from build123d import *

# Parameters (mm, degrees)
ESBO_O1_R                     = 7.5
RESSALTO_EXTRUS_O1_DEPTH      = 95
CORTE_EXTRUS_O1_START         = -7.5
ESBO_O2_R                     = 7.5
ESBO_O2_R_2                   = 6.5
CORTE_EXTRUS_O1_DEPTH         = 7.5
FILETE1_R                     = 5
FURO_ROSCADO_DE_M6X1_01_D     = 5
FURO_ROSCADO_DE_M6X1_01_DEPTH = 15.497848452
FURO_ROSCADO_DE_M6X1_01_TIP   = 1.502151548
CHANFRO1_SIZE                 = 0.5
CORTE_EXTRUS_O2_DEPTH         = 96.590271472
CORTE_EXTRUS_O2_DEPTH_BACK    = 96.590271472
ESBO_O8_W                     = 1
ESBO_O8_H                     = 50


with BuildPart() as part:
    # Esboço1 → Ressalto-extrusão1 (new, symmetric)
    with BuildSketch(Plane.XY):
        Circle(ESBO_O1_R)
    extrude(amount=RESSALTO_EXTRUS_O1_DEPTH, both=True)

    # Esboço2 → Corte-extrusão1 (cut)
    with BuildSketch(Plane(origin=(0, 0, -95), x_dir=(-1, 0, 0), z_dir=(0, 0, -1)).offset(CORTE_EXTRUS_O1_START)):
        Circle(ESBO_O2_R)
        Circle(ESBO_O2_R_2, mode=Mode.SUBTRACT)
    extrude(amount=CORTE_EXTRUS_O1_DEPTH, mode=Mode.SUBTRACT)

    # Filete1
    filete1_edges = [part.edges().sort_by_distance(p)[0] for p in [
        (-7.5, 0, 95),
    ]]
    fillet(filete1_edges, radius=FILETE1_R)

    # Furo roscado de M6x1.01
    with Locations(Plane(origin=(0, 0, -95), x_dir=(-1, 0, 0), z_dir=(0, 0, -1))):
        with Locations((0, 0)):
            Hole(FURO_ROSCADO_DE_M6X1_01_D / 2, depth=FURO_ROSCADO_DE_M6X1_01_DEPTH)
            with Locations((0, 0, -(FURO_ROSCADO_DE_M6X1_01_DEPTH + FURO_ROSCADO_DE_M6X1_01_TIP / 2))):  # 118° drill point
                Cone(0, FURO_ROSCADO_DE_M6X1_01_D / 2, FURO_ROSCADO_DE_M6X1_01_TIP, mode=Mode.SUBTRACT)

    # Chanfro1
    chanfro1_edges = [part.edges().sort_by_distance(p)[0] for p in [
        (6.5, 0, -95),
    ]]
    chamfer(chanfro1_edges, length=CHANFRO1_SIZE)

    # Esboço8 → Corte-extrusão2 (cut, two sides: drawn at the far end of the back side and taken through both)
    with BuildSketch(Plane(origin=(0, 0, 0), x_dir=(1, 0, 0), z_dir=(0, 1, 0)).offset(-CORTE_EXTRUS_O2_DEPTH_BACK)):
        with Locations((7, -45)):
            Rectangle(ESBO_O8_W, ESBO_O8_H)
    extrude(amount=CORTE_EXTRUS_O2_DEPTH + CORTE_EXTRUS_O2_DEPTH_BACK, mode=Mode.SUBTRACT)


solid = part.part
The listing builds one solid part. Answer for the finished solid, in the listing's coordinates (mm). A direction names the side the tool comes from. Round coordinates to 2 decimals unless told otherwise and drop trailing zeros. Order: outer loops, then holes, each group sorted by start corner. A loop starts at its lowest first (then second) coordinate and runs counter-clockwise, first axis right, second up. Notation, with made-up numbers: M -9.75,50 L 42.25,50 A17 cw 42.25,67 Z; hole C 41,48 d7. An arc over 180 degrees is marked long. Answer in a Markdown table with one row per item. Add a question column.
1) Determine the mould class of faces 4 (the face through (0, 0, -78)), 5 (the face through (-7.493, 0.33, 2.493)), 6 (the face through (-0.54, -2.44, -87.14)), 7 (the face through (3, 0, -95)) for opening direction X: pulls with the +X half, pulls with the -X half, needs draft (parallel to the pull), parting line crosses it, or undercut.
2) Flat-ended cylindrical pins translate along their axes: pin 1 Ø2 at (y, z) = (5, 14) entering from -X; pin 2 Ø3.5 at (y, z) = (0, 50) entering from +X; pin 3 Ø0.5 at (x, y) = (7, 0) entering from -Z. Find the tip coordinate at first contact, or state that the pin passes through.
3) Consider line 1 along Y through (x, z) = (0, -86.75); line 2 along X through (y, z) = (-4.5, 26); line 3 along Z through (x, y) = (-0.5, -2.75). Determine where each line is inside the solid, lowest interval first. Write a range as from..to.
4) The part is cut by section A-A on z = 30. Determine the outline of the cut face in (x, y).
5) Which of the six approach directions +Z, -Z, +X, -X, +Y, -Y give full straight-line access (tool end or side, diameter ignored) to faces 1 (the face through (0, 0, 95)), 2 (the face through (6, 3, -87.5)), 3 (the face through (6.5, 0, 45))?
Findings below:
| question | item | result |
|---|---|---|
| 1 | face 4 | undercut |
| 1 | face 5 | parting line crosses it |
| 1 | face 6 | undercut |
| 1 | face 7 | needs draft |
| 2 | pin 1 | stops at x = -6.34 |
| 2 | pin 2 | stops at x = 6.5 |
| 2 | pin 3 | stops at z = -87.5 |
| 3 | line 1 | y = -7.5..-2.5, 2.5..7.5 |
| 3 | line 2 | x = -6..6 |
| 3 | line 3 | z = -95..94.99 |
| 4 | outline | M 6.5,-3.74 L 6.5,3.74 A7.5 ccw long Z |
| 5 | face 1 | +Z, +X, -X, +Y, -Y |
| 5 | face 2 | -Z |
| 5 | face 3 | +X, +Y, -Y |
